Drawing for the job (mm, zero at the part's lowest x, y, z). Round coordinates to 2 decimals unless told otherwise and drop trailing zeros. Write each loop counter-clockwise with the first axis right and the second up, starting at its lowest first coordinate (ties: lowest second). Pieces come first, ordered by that corner, then holes. Notation, with made-up numbers: (61.25, 10.25) - (119.25, 10.25) arc R13 ccw to (119.25, 17.25) - close; hole circle Ø8 at (-13, 45.25). An arc over 180 degrees is marked (long way). One line per question, with ' | ' between items.
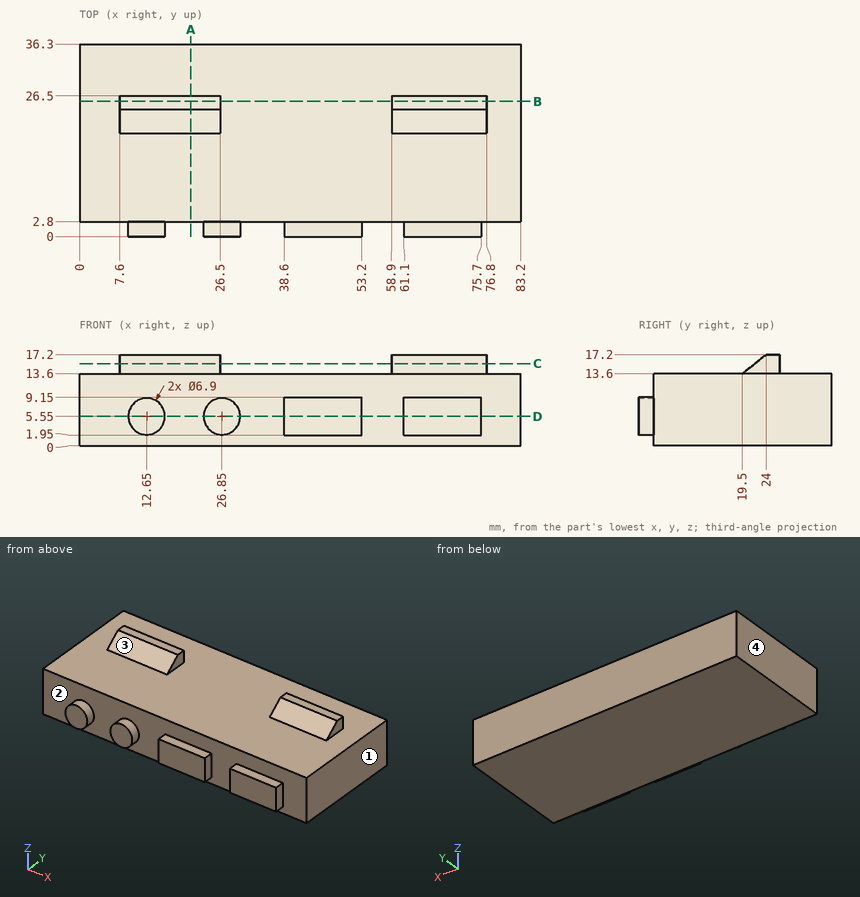
Q1. Saw through at A-A, the plane x = 21. List the corners of the cut face in (y, z).
Found:
outline: (2.8, 0) - (36.3, 0) - (36.3, 13.6) - (26.5, 13.6) - (26.5, 17.2) - (24, 17.2) - (19.5, 13.6) - (2.8, 13.6) - close
Q2. Saw through at D-D, the plane z = 5.55. List the corners of the cut face in (x, y).
Found:
outline: (0, 2.8) - (9.2, 2.8) - (9.2, 0) - (16.1, 0) - (16.1, 2.8) - (23.4, 2.8) - (23.4, 0) - (30.3, 0) - (30.3, 2.8) - (38.6, 2.8) - (38.6, 0) - (53.2, 0) - (53.2, 2.8) - (61.1, 2.8) - (61.1, 0) - (75.7, 0) - (75.7, 2.8) - (83.2, 2.8) - (83.2, 36.3) - (0, 36.3) - close
Q3. Pull direction X, two halves, no side cores. Call the marked faces 1, 2, 3 and 4: +X half, -X half, draft (parallel to the pull), parting line (faces both ways), or undercut.
Found:
face 1: +X half | face 2: undercut | face 3: draft | face 4: -X half
Q4. Saw through at C-C, the plane z = 15.5. List the corners of the cut face in (x, y) (3 decimals), then the cut area to 3 significant figures.
Found:
outline: (7.6, 21.875) - (26.5, 21.875) - (26.5, 26.5) - (7.6, 26.5) - close; (58.9, 21.875) - (76.8, 21.875) - (76.8, 26.5) - (58.9, 26.5) - close | area: 170 mm^2
Q5. Drop flat-ended pins along their axis: pin 1 (5 mm diameter, centred on x = 47.5, y = 15.5, fed in from +Z); pin 2 (1.4 mm diameter, centred on x = 49, y = 2, fed in from -Z); pin 3 (1.8 mm diameter, centred on y = 22, z = 15.5, fed in from -X). Give the stop position or say it passes through.
Found:
pin 1: z = 13.6 | pin 2: z = 1.95 | pin 3: x = 7.6
Q6. Saw through at B-B, the plane y = 25.5. List the corners of the cut face in (x, z).
Found:
outline: (0, 0) - (83.2, 0) - (83.2, 13.6) - (76.8, 13.6) - (76.8, 17.2) - (58.9, 17.2) - (58.9, 13.6) - (26.5, 13.6) - (26.5, 17.2) - (7.6, 17.2) - (7.6, 13.6) - (0, 13.6) - close
Q7. Drill centre lines: L1, parallel to Z at x = 70.5, y = 15; L2, parallel to Y at x = 6.5, z = 1.25; L3, parallel to Y at x = 72.5, z = 16.25. Where is each one in solid material? Low to high. Write a range as from..to.
Found:
L1: 0..13.6 | L2: 2.8..36.3 | L3: 22.81..26.5
